```python
from build123d import *

# Parameters (mm, degrees)
RESSALTO_EXTRUS_O1_DEPTH = 2


with BuildPart() as part:
    # Esboço1 → Ressalto-extrusão1 (new body)
    with BuildSketch(Plane(origin=(0, 0, 0), x_dir=(1, 0, 0), z_dir=(0, 1, 0))):
        with BuildLine():
            Line((-23.5, 14.5), (-23.5, -7.5))
            ThreePointArc((-23.5, -7.5), (-20.571067812, -14.571067812), (-13.5, -17.5))
            Line((-13.5, -17.5), (13.5, -17.5))
            ThreePointArc((13.5, -17.5), (20.571067812, -14.571067812), (23.5, -7.5))
            Line((23.5, -7.5), (23.5, 14.5))
            ThreePointArc((23.5, 14.5), (23.207106781, 15.207106781), (22.5, 15.5))
            Line((22.5, 15.5), (20, 15.5))
            ThreePointArc((20, 15.5), (19.292893219, 15.207106781), (19, 14.5))
            Line((19, 14.5), (19, 4))
            ThreePointArc((19, 4), (16.5, 1.5), (14, 4))
            Line((14, 4), (14, 16.5))
            ThreePointArc((14, 16.5), (13.707106781, 17.207106781), (13, 17.5))
            Line((13, 17.5), (-13, 17.5))
            ThreePointArc((-13, 17.5), (-13.707106781, 17.207106781), (-14, 16.5))
            Line((-14, 16.5), (-14, 4))
            ThreePointArc((-14, 4), (-16.5, 1.5), (-19, 4))
            Line((-19, 4), (-19, 14.5))
            ThreePointArc((-19, 14.5), (-19.292893219, 15.207106781), (-20, 15.5))
            Line((-20, 15.5), (-22.5, 15.5))
            ThreePointArc((-22.5, 15.5), (-23.207106781, 15.207106781), (-23.5, 14.5))
        make_face()
    extrude(amount=RESSALTO_EXTRUS_O1_DEPTH)


solid = part.part
```
The listing builds one solid part. Answer for the finished solid, in the listing's coordinates (mm). A direction names the side the tool comes from. Coordinates: 2 decimals unless noted, no trailing zeros. Write each loop counter-clockwise with the first axis right and the second up, starting at its lowest first coordinate (ties: lowest second). Pieces come first, ordered by that corner, then holes. Notation, with made-up numbers: M 60.5,-39.5 L 76.5,-39.5 A20 ccw 76.5,-12.5 Z; hole C 8,25.25 d9. An arc over 180 degrees is marked long. Use a Markdown table: item, result. Add a question column.
1. Straight lines are drawn through the part: line 1 along X through (y, z) = (1.1, -4); line 2 along X through (y, z) = (0.4, -15); line 3 along X through (y, z) = (1.2, 10.5). For each, find the intervals that lie inside material, in ascending order. Write a range as [from, to].
2. Section C-C (x = -16.5) is taken. Give the vertices of the cut face in (y, z), plus the area to 3 significant figures.
3. Given P1, Ø0.6, axis at x = -21, y = 1, coming from the -Z side, flat-ended and moving along its own axis, determine where the tip first touches the part or whether it passes through.
4. Which of the six approach directions +Z, -Z, +X, -X, +Y, -Y give full straight-line access (tool end or side, diameter ignored) to faces 1 (the flat face through (-21, 1, -15.5)), 2 (the flat face through (21, 1, -15.5)), 3 (the flat face through (-19, 1, -9))?
5. Section D-D (z = 12) is taken. Give the vertices of the cut face in (x, y), plus the area to 3 significant figures.
6. Section B-B (y = 1.4) is taken. Give the vertices of the cut face in (x, z), plus the area to 3 significant figures.
7. Section A-A (z = -4.5) is taken. Give the vertices of the cut face in (x, y).
8. For a pull along X with two mould halves and no side action, classify faces 4 (the flat face through (14, 1, -10)), 5 (the flat face through (23.5, 1, -3)), 6 (the cylindrical face through (-20.65, 0.99, 14.49)), 7 (the cylindrical face through (19.301, 0.986, -15.215)) as +X half, -X half, draft (parallel to the pull), parting line (faces both ways), or undercut.
Data:
| question | item | result |
|---|---|---|
| 1 | line 1 | x = [-23.5, -19], [-14, 14], [19, 23.5] |
| 1 | line 2 | x = [-23.37, -19.13], [-14, 14], [19.13, 23.37] |
| 1 | line 3 | x = [-23.04, 23.04] |
| 2 | outline | M 0,-1.5 L 2,-1.5 L 2,17.04 L 0,17.04 Z |
| 2 | area | 37.1 mm2 |
| 3 | P1 | stops at z = -15.5 |
| 4 | face 1 | -Z, -X, +Y, -Y |
| 4 | face 2 | -Z, +X, +Y, -Y |
| 4 | face 3 | -Z, +Y, -Y |
| 5 | outline | M -22.43,0 L 22.43,0 L 22.43,2 L -22.43,2 Z |
| 5 | area | 89.7 mm2 |
| 6 | outline | M -23.5,-14.5 A1 ccw -22.5,-15.5 L -20,-15.5 A1 ccw -19,-14.5 L -19,-4 A2.5 cw -14,-4 L -14,-16.5 A1 ccw -13,-17.5 L 13,-17.5 A1 ccw 14,-16.5 L 14,-4 A2.5 cw 19,-4 L 19,-14.5 A1 ccw 20,-15.5 L 22.5,-15.5 A1 ccw 23.5,-14.5 L 23.5,7.5 A10 ccw 13.5,17.5 L -13.5,17.5 A10 ccw -23.5,7.5 Z |
| 6 | area | 1,430 mm2 |
| 7 | outline | M -23.5,0 L -19,0 L -19,2 L -23.5,2 Z; M -14,0 L 14,0 L 14,2 L -14,2 Z; M 19,0 L 23.5,0 L 23.5,2 L 19,2 Z |
| 8 | face 4 | undercut |
| 8 | face 5 | +X half |
| 8 | face 6 | -X half |
| 8 | face 7 | undercut |
